from build123d import *

# Parameters (mm, degrees)
SKETCH1_R           = 2.5
BOSS_EXTRUDE2_DEPTH = 3
SKETCH2_R           = 2.3
BOSS_EXTRUDE3_DEPTH = 4
SKETCH3_R           = 2.7
BOSS_EXTRUDE4_DEPTH = 1
CHAMFER1_SIZE       = 0.4
SKETCH4_R           = 2.05
BOSS_EXTRUDE5_DEPTH = 0.65
CHAMFER2_SIZE       = 0.65
CUT_EXTRUDE1_REACH  = 75.679
SKETCH7_R           = 1.2
CUT_EXTRUDE2_DEPTH  = 5.65
CHAMFER3_SIZE       = 0.7


with BuildPart() as part:
    # Sketch1 → Boss-Extrude2 (new body)
    with BuildSketch(Plane(origin=(0, 0, 0), x_dir=(1, 0, 0), z_dir=(0, 1, 0))):
        with BuildLine():
            ThreePointArc((-6.116355206, -22.650875646), (-26.749356674, -15.248026431), (-40.382392076, 1.917732271))
            ThreePointArc((-40.382392076, 1.917732271), (-44.99801909, 4.999999608), (-49.616086933, 1.921390494))
            ThreePointArc((-49.616086933, 1.921390494), (-53.104028793, -5.679123666), (-55.276433102, -13.75465544))
            ThreePointArc((-55.276433102, -13.75465544), (-55.245679697, -13.416577441), (-55.192056675, -13.081365453))
            ThreePointArc((-55.192056675, -13.081365453), (-52.322107352, -33.280314666), (-37.56541985, -47.368406531))
            ThreePointArc((-37.56541985, -47.368406531), (-18.529366308, -39.223016825), (-6.116355206, -22.650875646))
        make_face()
        with Locations(Location((-45, 0, 0), (0, 0, 270))):
            Circle(SKETCH1_R, mode=Mode.SUBTRACT)
    extrude(amount=-BOSS_EXTRUDE2_DEPTH)

    # Sketch2 → Boss-Extrude3 (add)
    with BuildSketch(Plane(origin=(0, 0, 0), x_dir=(1, 0, 0), z_dir=(0, 1, 0))):
        with Locations(Location((-50.284485705, -14.03831225, 0), (0, 0, 270))):
            Circle(SKETCH2_R)
    extrude(amount=BOSS_EXTRUDE3_DEPTH)

    # Sketch3 → Boss-Extrude4 (add)
    with BuildSketch(Plane(origin=(0, 4, 0), x_dir=(1, 0, 0), z_dir=(0, 1, 0))):
        with Locations(Location((-50.284485705, -14.03831225, 0), (0, 0, 270))):
            Circle(SKETCH3_R)
    extrude(amount=BOSS_EXTRUDE4_DEPTH)

    # Chamfer1
    chamfer1_edges = [part.edges().sort_by_distance(p)[0] for p in [
        (-50.284485705, 4, 11.73831225),
    ]]
    chamfer(chamfer1_edges, length=CHAMFER1_SIZE - 0.0001)  # a hair under: the kernel refuses the full size

    # Sketch4 → Boss-Extrude5 (add)
    with BuildSketch(Plane(origin=(0, 5, 0), x_dir=(1, 0, 0), z_dir=(0, 1, 0))):
        with Locations(Location((-50.284485705, -14.03831225, 0), (0, 0, 270))):
            Circle(SKETCH4_R)
    extrude(amount=BOSS_EXTRUDE5_DEPTH)

    # Chamfer2
    chamfer2_edges = [part.edges().sort_by_distance(p)[0] for p in [
        (-50.284485705, 5, 11.98831225),
    ]]
    chamfer(chamfer2_edges, length=CHAMFER2_SIZE - 0.0001)  # a hair under: the kernel refuses the full size

    # Cut-Extrude1: up to this face of the body (flat: up to its plane)
    cut_extrude1_end = Plane(part.part.faces().sort_by_distance((-35.615181699, 0, 24.623132095))[0])
    # Sketch6 → Cut-Extrude1 (cut, up to the picked face)
    with BuildSketch(Plane(origin=(0, 5.65, 0), x_dir=(1, 0, 0), z_dir=(0, 1, 0)), mode=Mode.PRIVATE) as cut_extrude1_sk1:
        with BuildLine():
            Line((-50.254713835, -16.088096052), (-48.910426349, -12.516977019))
            ThreePointArc((-48.910426349, -12.516977019), (-49.562272658, -12.119742909), (-50.314257574, -11.988528448))
            Line((-50.314257574, -11.988528448), (-51.65854506, -15.559647482))
            ThreePointArc((-51.65854506, -15.559647482), (-51.006698751, -15.956881591), (-50.254713835, -16.088096052))
        make_face()
    cut_extrude1_tool1 = split(extrude(cut_extrude1_sk1.sketch, amount=-CUT_EXTRUDE1_REACH, mode=Mode.PRIVATE), bisect_by=cut_extrude1_end, keep=Keep.BOTH, mode=Mode.PRIVATE)
    # Sketch6 → Cut-Extrude1 (cut, up to the picked face)
    with BuildSketch(Plane(origin=(0, 5.65, 0), x_dir=(1, 0, 0), z_dir=(0, 1, 0)), mode=Mode.PRIVATE) as cut_extrude1_sk2:
        with BuildLine():
            Line((-48.910426349, -12.516977019), (-47.84100442, -9.676042289))
            ThreePointArc((-47.84100442, -9.676042289), (-48.52299047, -9.358874834), (-49.244835645, -9.147593719))
            Line((-49.244835645, -9.147593719), (-50.314257574, -11.988528448))
            ThreePointArc((-50.314257574, -11.988528448), (-49.562272658, -12.119742909), (-48.910426349, -12.516977019))
        make_face()
    cut_extrude1_tool2 = split(extrude(cut_extrude1_sk2.sketch, amount=-CUT_EXTRUDE1_REACH, mode=Mode.PRIVATE), bisect_by=cut_extrude1_end, keep=Keep.BOTH, mode=Mode.PRIVATE)
    # Sketch6 → Cut-Extrude1 (cut, up to the picked face)
    with BuildSketch(Plane(origin=(0, 5.65, 0), x_dir=(1, 0, 0), z_dir=(0, 1, 0)), mode=Mode.PRIVATE) as cut_extrude1_sk3:
        with BuildLine():
            Line((-51.324135764, -18.929030782), (-50.254713835, -16.088096052))
            ThreePointArc((-50.254713835, -16.088096052), (-51.006698751, -15.956881591), (-51.65854506, -15.559647482))
            Line((-51.65854506, -15.559647482), (-52.727966989, -18.400582211))
            ThreePointArc((-52.727966989, -18.400582211), (-52.04598094, -18.717749667), (-51.324135764, -18.929030782))
        make_face()
    cut_extrude1_tool3 = split(extrude(cut_extrude1_sk3.sketch, amount=-CUT_EXTRUDE1_REACH, mode=Mode.PRIVATE), bisect_by=cut_extrude1_end, keep=Keep.BOTH, mode=Mode.PRIVATE)
    # Sketch6 → Cut-Extrude1 (cut, up to the picked face)
    with BuildSketch(Plane(origin=(0, 5.65, 0), x_dir=(1, 0, 0), z_dir=(0, 1, 0)), mode=Mode.PRIVATE) as cut_extrude1_sk4:
        with BuildLine():
            Line((-48.910426349, -12.516977019), (-47.84100442, -9.676042289))
            ThreePointArc((-47.84100442, -9.676042289), (-48.52299047, -9.358874834), (-49.244835645, -9.147593719))
            Line((-49.244835645, -9.147593719), (-50.314257574, -11.988528448))
            ThreePointArc((-50.314257574, -11.988528448), (-49.562272658, -12.119742909), (-48.910426349, -12.516977019))
        make_face()
    cut_extrude1_tool4 = split(extrude(cut_extrude1_sk4.sketch, amount=-CUT_EXTRUDE1_REACH, mode=Mode.PRIVATE), bisect_by=cut_extrude1_end, keep=Keep.BOTH, mode=Mode.PRIVATE)
    # Sketch6 → Cut-Extrude1 (cut, up to the picked face)
    with BuildSketch(Plane(origin=(0, 5.65, 0), x_dir=(1, 0, 0), z_dir=(0, 1, 0)), mode=Mode.PRIVATE) as cut_extrude1_sk5:
        with BuildLine():
            Line((-51.324135764, -18.929030782), (-50.254713835, -16.088096052))
            ThreePointArc((-50.254713835, -16.088096052), (-51.006698751, -15.956881591), (-51.65854506, -15.559647482))
            Line((-51.65854506, -15.559647482), (-52.727966989, -18.400582211))
            ThreePointArc((-52.727966989, -18.400582211), (-52.04598094, -18.717749667), (-51.324135764, -18.929030782))
        make_face()
    cut_extrude1_tool5 = split(extrude(cut_extrude1_sk5.sketch, amount=-CUT_EXTRUDE1_REACH, mode=Mode.PRIVATE), bisect_by=cut_extrude1_end, keep=Keep.BOTH, mode=Mode.PRIVATE)
    add(cut_extrude1_tool1.solids().sort_by(Axis((-50.284486, 5.65, 14.038312), (0, -1, 0)))[0], mode=Mode.SUBTRACT)
    add(cut_extrude1_tool2.solids().sort_by(Axis((-49.05426, 5.65, 10.770199), (0, -1, 0)))[0], mode=Mode.SUBTRACT)
    add(cut_extrude1_tool3.solids().sort_by(Axis((-51.514712, 5.65, 17.306426), (0, -1, 0)))[0], mode=Mode.SUBTRACT)
    add(cut_extrude1_tool4.solids().sort_by(Axis((-49.05426, 5.65, 10.770199), (0, -1, 0)))[0], mode=Mode.SUBTRACT)
    add(cut_extrude1_tool5.solids().sort_by(Axis((-51.514712, 5.65, 17.306426), (0, -1, 0)))[0], mode=Mode.SUBTRACT)

    # Sketch7 → Cut-Extrude2 (cut)
    with BuildSketch(Plane(origin=(0, 5.65, 0), x_dir=(1, 0, 0), z_dir=(0, 1, 0))):
        with Locations((-50.284485705, -14.03831225)):
            Circle(SKETCH7_R)
    extrude(amount=-CUT_EXTRUDE2_DEPTH, mode=Mode.SUBTRACT)

    # Chamfer3
    chamfer3_edges = [part.edges().sort_by_distance(p)[0] for p in [
        (-45, 0, -2.5),
    ]]
    chamfer(chamfer3_edges, length=CHAMFER3_SIZE)


solid = part.part
Geometry: final body of the model. Coordinates: model frame, mm. Round coordinates to 2 decimals unless told otherwise and drop trailing zeros. Loops run counter-clockwise (first coordinate to the right, second up) from the corner with the lowest first, then second, coordinate; pieces in that order, holes last.
Q1. Section C-C on x = -45. Return loops of the section in (y, z), plus the area to 3 significant figures.
Q2. Pull-direction query (X, two-part tool) for faces 1 (the cylindrical face through (-51.4, 2.9, 13.6)), 2 (the cylindrical face through (-52.454, -1.479, 33.021)), 3 (the flat face through (-37, -3, 27)); classes: released by +X, released by -X, zero draft, split by the parting line, or undercut.
Q3. Material intervals for L1, parallel to Y at x = -18, z = 25; L2, parallel to X at y = -1.7, z = 0; L3, parallel to X at y = -0.25, z = 12, sorted ascending.
Q4. Pin query (flat end, axial travel): P1, Ø6, axis at x = -37.5, z = 41, coming from the +Y side; P2, Ø3, axis at y = -0.5, z = 3, coming from the -X side; P3, Ø1.5, axis at y = 2.5, z = 11.5, coming from the -X side. Return the tip coordinate at first contact, or that it passes through.
Q5. Section D-D on y = 2.5. Return loops of the section in (x, z), plus the area to 3 significant figures.
Q6. Section B-B on y = -1.75. Return loops of the section in (x, z).
Q7. Section A-A on z = 0. Return loops of the section in (x, y), plus the area to 3 significant figures.
Evaluation:
1. outline: (-3, -5) - (0, -5) - (0, -3.2) - (-0.7, -2.5) - (-3, -2.5) - close; (-3, 2.5) - (-0.7, 2.5) - (0, 3.2) - (0, 42.59) - (-3, 42.59) - close
1. area: 127 mm2
2. face 1: undercut
2. face 2: released by -X
2. face 3: zero draft
3. L1: y = -3 to 0
3. L2: x = -50.65 to -47.5, -42.5 to -39.53
3. L3: x = -54.93 to -30.72
4. P1: stops at y = 0
4. P2: stops at x = -52.66
4. P3: stops at x = -51.73
5. outline: (-51.75, 15.81) arc R2.3 ccw to (-50.22, 11.74) - (-50.66, 12.9) arc R1.2 cw to (-51.32, 14.65) - close; (-50.35, 16.34) - (-49.91, 15.18) arc R1.2 cw to (-49.25, 13.43) - (-48.82, 12.27) arc R2.3 ccw to start
5. area: 8.67 mm2
6. outline: (-55.28, 13.75) arc R50 ccw to (-49.62, -1.92) arc R5 ccw to (-40.38, -1.92) arc R40 cw to (-6.12, 22.65) arc R40 ccw to (-37.57, 47.37) arc R31.14 ccw to (-55.19, 13.08) arc R5 cw to start; hole circle Ø5 at (-45, 0)
7. outline: (-50.65, -3) - (-47.5, -3) - (-47.5, -0.7) - (-48.2, 0) - (-50.65, 0) - close; (-42.5, -3) - (-39.53, -3) - (-39.53, 0) - (-41.8, 0) - (-42.5, -0.7) - close
7. area: 17.9 mm2
